For this review, take the finished solid that the model builds, in its own axes (mm). A direction names the side the tool comes from. Round coordinates to 2 decimals unless told otherwise and drop trailing zeros. Order: outer loops, then holes, each group sorted by start corner. A loop starts at its lowest first (then second) coordinate and runs counter-clockwise, first axis right, second up. Notation, with made-up numbers: (2, -15) -> (29, -15) arc R17 cw to (29, -5) -> close; hole circle Ø8 at (-40, 59). An arc over 180 degrees is marked (long way). Use a Markdown table: item, result. Add a question column.
1) Clearance check with flat-ended pins moving along their axes: P1, Ø7.5, axis at x = -22, y = -5, coming from the +Z side; P2, Ø3, axis at x = -6.5, y = -4.5, coming from the +Z side; P3, Ø1, axis at y = 10.5, z = -4, coming from the -X side; P4, Ø3, axis at y = -3, z = -4, coming from the -X side. State where each tip first meets the part, or that it passes through.
2) Consider section B-B (y = 21.5). State the section outline as (x, z) points, plus the area to 3 significant figures.
3) Wall thickness on line 1 along X through (y, z) = (11.5, -4.5); line 2 along Y through (x, z) = (8.3, 0); line 3 along Z through (x, y) = (-20, 21.5): over which ranges is each line inside the solid? List them lowest first. Write a range as [from, to].
4) Consider section A-A (y = 11). State the section outline as (x, z) points.
5) Draft analysis for pull direction Z (two halves, no side actions). For faces 5 (the face through (-7.5, 15, -4)), 6 (the face through (8.6, -18.8, -1.6)), 7 (the face through (-18, -1, 3.5)), state which applies: pulls with the +Z half, pulls with the -Z half, needs draft (parallel to the pull), parting line crosses it, or undercut.
6) Machinability: for faces 1 (the face through (1.4, 2.5, -4.5)), 2 (the face through (-16, 10, 4)), 3 (the face through (-26, 18, -3.5)), 4 (the face through (-18, -4, -3.5)), which of the approach directions +Z, -Z, +X, -X, +Y, -Y give a long, thin tool a straight path to every point of the face, cutting with its end or side? Answer none if there is none.
7) Consider section C-C (x = 3). State the section outline as (y, z) points, plus the area to 3 significant figures.
8) Consider section D-D (z = -6.25). State the section outline as (x, y) points, plus the area to 3 significant figures.
```python
from build123d import *

# Parameters (mm, degrees)
SKETCH2_R               = 10
BOSS_EXTRUDE1_DEPTH     = 30
CUT_EXTRUDE1_START      = -10
SKETCH3_R               = 10
SKETCH3_R_2             = 7.5
CUT_EXTRUDE1_DEPTH      = 10
CUT_EXTRUDE3_DEPTH      = 10
CUT_EXTRUDE3_DEPTH_BACK = 10
SKETCH5_R               = 2
FILLET2_R               = 10
BOSS_EXTRUDE2_START     = -67.5
SKETCH7_R               = 10
BOSS_EXTRUDE2_DEPTH     = 67.5
SKETCH8_R               = 50
SKETCH8_R_2             = 10
CUT_EXTRUDE6_DEPTH      = 107.770782567
SKETCH9_R               = 7.5
CUT_EXTRUDE7_DEPTH      = 10
CUT_EXTRUDE8_DEPTH      = 10
CUT_EXTRUDE8_DEPTH_BACK = 10
SKETCH10_R              = 2
CUT_EXTRUDE9_DEPTH      = 48
CUT_EXTRUDE9_DEPTH_BACK = 29
SKETCH12_W              = 23.028444079
SKETCH12_H              = 65
SKETCH13_W              = 45
SKETCH13_H              = 7
BOSS_EXTRUDE3_DEPTH     = 15
SKETCH14_W              = 7
SKETCH14_H              = 25.920736851
BOSS_EXTRUDE4_DEPTH     = 2
SKETCH15_W              = 17.5
SKETCH15_H              = 25.366229316
BOSS_EXTRUDE5_DEPTH     = 2
SKETCH15_W_2            = 16.786959534
BOSS_EXTRUDE5_2_DEPTH   = 2
BOSS_EXTRUDE6_START     = -44.28696
BOSS_EXTRUDE6_DEPTH     = 44.28696
SKETCH17_W              = 10
SKETCH17_H              = 2
SKETCH17_W_2            = 18.286959534
SKETCH17_W_3            = 19
CUT_EXTRUDE10_DEPTH     = 8
BOSS_EXTRUDE7_DEPTH     = 19.367497
CUT_EXTRUDE11_DEPTH     = 8
SKETCH22_W              = 1.1
SKETCH22_H              = 2
CUT_EXTRUDE12_DEPTH     = 32
SKETCH23_W              = 5.9
SKETCH23_H              = 12.960368426
CUT_EXTRUDE13_DEPTH     = 10


with BuildPart() as part:
    # Sketch1 → Revolve1 (revolve)
    with BuildSketch(Plane.XY):
        Polygon((50, 25), (0, 25), (0, 22.5), (45, 22.5), (45, -22.5), (0, -22.5), (0, -25), (50, -25), align=None)
    revolve(axis=Axis((0, -25, 0), (0, 1, 0)))

    # Sketch2 → Boss-Extrude1 (add)
    with BuildSketch(Plane(origin=(0, 25, 0), x_dir=(1, 0, 0), z_dir=(0, 1, 0))):
        with Locations(Location((0, 0, 0), (0, 0, 180))):
            Circle(SKETCH2_R)
    extrude(amount=BOSS_EXTRUDE1_DEPTH)

    # Sketch3 → Cut-Extrude1 (cut)
    with BuildSketch(Plane(origin=(0, 55, 0), x_dir=(1, 0, 0), z_dir=(0, 1, 0)).offset(CUT_EXTRUDE1_START)):
        with Locations(Location((0, 0, 0), (0, 0, 180))):
            Circle(SKETCH3_R)
        with Locations(Location((0, 0, 0), (0, 0, 180))):
            Circle(SKETCH3_R_2, mode=Mode.SUBTRACT)
    extrude(amount=CUT_EXTRUDE1_DEPTH, mode=Mode.SUBTRACT)

    # Sketch5 → Cut-Extrude3 (cut, two sides: drawn at the far end of the back side and taken through both)
    with BuildSketch(Plane(origin=(0, 0, 0), x_dir=(0, 0, -1), z_dir=(1, 0, 0)).offset(-CUT_EXTRUDE3_DEPTH_BACK)):
        with Locations(Location((0, 50, 0), (0, 0, 180))):
            Circle(SKETCH5_R)
    extrude(amount=CUT_EXTRUDE3_DEPTH + CUT_EXTRUDE3_DEPTH_BACK, mode=Mode.SUBTRACT)

    # Fillet2
    fillet2_edges = [part.edges().sort_by_distance(p)[0] for p in [
        (-50, 25, 0),
    ]]
    fillet(fillet2_edges, radius=FILLET2_R)

    # Sketch7 → Boss-Extrude2 (add)
    with BuildSketch(Plane(origin=(0, 45, 0), x_dir=(1, 0, 0), z_dir=(0, 1, 0)).offset(BOSS_EXTRUDE2_START)):
        with Locations(Location((0, 0, 0), (0, 0, 180))):
            Circle(SKETCH7_R)
    extrude(amount=BOSS_EXTRUDE2_DEPTH)

    # Sketch8 → Cut-Extrude6 (cut, through all)
    with BuildSketch(Plane(origin=(0, 55, 0), x_dir=(1, 0, 0), z_dir=(0, 1, 0))):
        Circle(SKETCH8_R)
        with Locations(Location((0, 0, 0), (0, 0, 180))):
            Circle(SKETCH8_R_2, mode=Mode.SUBTRACT)
    extrude(amount=-CUT_EXTRUDE6_DEPTH, mode=Mode.SUBTRACT)

    # Sketch9 → Cut-Extrude7 (cut)
    with BuildSketch(Plane.XZ.offset(25)):
        with Locations(Location((0, 0, 0), (0, 0, 180))):
            Circle(SKETCH9_R)
    extrude(amount=-CUT_EXTRUDE7_DEPTH, mode=Mode.SUBTRACT)

    # Sketch10 → Cut-Extrude8 (cut, two sides: drawn at the far end of the back side and taken through both)
    with BuildSketch(Plane(origin=(0, 0, 0), x_dir=(0, 0, -1), z_dir=(1, 0, 0)).offset(-CUT_EXTRUDE8_DEPTH_BACK)):
        with Locations(Location((0, -20, 0), (0, 0, 180))):
            Circle(SKETCH10_R)
    extrude(amount=CUT_EXTRUDE8_DEPTH + CUT_EXTRUDE8_DEPTH_BACK, mode=Mode.SUBTRACT)

    # Sketch12 → Cut-Extrude9 (cut, two sides: drawn at the far end of the back side and taken through both)
    with BuildSketch(Plane(origin=(0, 0, 0), x_dir=(0, 0, -1), z_dir=(1, 0, 0)).offset(-CUT_EXTRUDE9_DEPTH_BACK)):
        with Locations((0.475794299, 22.5)):
            Rectangle(SKETCH12_W, SKETCH12_H)
    extrude(amount=CUT_EXTRUDE9_DEPTH + CUT_EXTRUDE9_DEPTH_BACK, mode=Mode.SUBTRACT)

    # Sketch13 → Boss-Extrude3 (add)
    with BuildSketch(Plane(origin=(0, -10, 0), x_dir=(1, 0, 0), z_dir=(0, 1, 0))):
        with Locations((-12.5, 0)):
            Rectangle(SKETCH13_W, SKETCH13_H)
    extrude(amount=BOSS_EXTRUDE3_DEPTH)

    # Sketch14 → Boss-Extrude4 (add)
    with BuildSketch(Plane.XY.offset(3.5)):
        with Locations((-12.5, 17.264610389)):
            Rectangle(SKETCH14_W, SKETCH14_H)
    extrude(amount=BOSS_EXTRUDE4_DEPTH)



with BuildPart() as body_2:
    # Sketch15 → Boss-Extrude5 (new body)
    with BuildSketch(Plane(origin=(0, 0, -3.5), x_dir=(-1, 0, 0), z_dir=(0, 0, -1))):
        with Locations((-1.25, 17.683114658)):
            Rectangle(SKETCH15_W, SKETCH15_H)
    extrude(amount=BOSS_EXTRUDE5_DEPTH)


with BuildPart() as body_3:
    # Sketch15 → Boss-Extrude5 2 (new body)
    with BuildSketch(Plane(origin=(0, 0, -3.5), x_dir=(-1, 0, 0), z_dir=(0, 0, -1))):
        with Locations((25.893479767, 17.683114658)):
            Rectangle(SKETCH15_W_2, SKETCH15_H)
    extrude(amount=BOSS_EXTRUDE5_2_DEPTH)


with BuildPart() as part_1:
    add(part.part)

    add(body_2.part)  # Boss-Extrude6 merges body 2

    add(body_3.part)  # Boss-Extrude6 merges body 3
    # Sketch16 → Boss-Extrude6 (add)
    with BuildSketch(Plane.ZY.offset(34.286959534).offset(BOSS_EXTRUDE6_START)):
        Polygon((-5.5, 5), (-3.5, 0), (-3.5, 5), align=None)
        Polygon((3.5, 0), (5.5, 4.304241963), (3.5, 4.304241963), align=None)
    extrude(amount=BOSS_EXTRUDE6_DEPTH)

    # Sketch17 → Cut-Extrude10 (cut)
    with BuildSketch(Plane(origin=(0, 5, 0), x_dir=(1, 0, 0), z_dir=(0, 1, 0))):
        with Locations((-12.5, 4.5)):
            Rectangle(SKETCH17_W, SKETCH17_H)
        with Locations((-25.143479767, -4.5)):
            Rectangle(SKETCH17_W_2, SKETCH17_H)
        with Locations((0.5, -4.5)):
            Rectangle(SKETCH17_W_3, SKETCH17_H)
    extrude(amount=-CUT_EXTRUDE10_DEPTH, mode=Mode.SUBTRACT)

    # Sketch18 → Boss-Extrude7 (add)
    with BuildSketch(Plane(origin=(10, 0, 0), x_dir=(0, 0, -1), z_dir=(1, 0, 0))):
        Polygon((-10, -10), (-3.5, -10), (-3.5, -2.5), align=None)
        Polygon((10, -10), (3.5, -4.366666667), (3.5, -10), align=None)
    extrude(amount=-BOSS_EXTRUDE7_DEPTH)

    # Sketch19 → Cut-Extrude11 (cut)
    with BuildSketch(Plane.XZ.offset(10)):
        with BuildLine():
            ThreePointArc((0, 10), (7.071067812, 7.071067812), (10, 0))
            Line((10, 0), (10, 10))
            Line((10, 10), (0, 10))
        make_face()
        with BuildLine():
            Line((-13.702189606, 3.5), (-9.367496998, 3.5))
            ThreePointArc((-9.367496998, 3.5), (-5.700877125, 8.215838363), (0, 10))
            Line((0, 10), (10, 10))
            ThreePointArc((10, 10), (-3.740194109, 13.638583065), (-13.702189606, 3.5))
        make_face()
        with BuildLine():
            ThreePointArc((10, 0), (1.778346145, -9.840603893), (-9.367496998, -3.5))
            Line((-9.367496998, -3.5), (-13.702189606, -3.5))
            ThreePointArc((-13.702189606, -3.5), (6.999217954, -12.288651188), (10, 10))
            Line((10, 10), (10, 0))
        make_face()
    extrude(amount=-CUT_EXTRUDE11_DEPTH, mode=Mode.SUBTRACT)

    # Sketch22 → Cut-Extrude12 (cut)
    with BuildSketch(Plane(origin=(0, 30.224978814, 0), x_dir=(1, 0, 0), z_dir=(0, 1, 0))):
        with Locations((-9.55, -4.5)):
            Rectangle(SKETCH22_W, SKETCH22_H)
    extrude(amount=-CUT_EXTRUDE12_DEPTH, mode=Mode.SUBTRACT)

    # Sketch23 → Cut-Extrude13 (cut)
    with BuildSketch(Plane.XY.offset(5.5)):
        with Locations((-13.05, 23.744794601)):
            Rectangle(SKETCH23_W, SKETCH23_H)
    extrude(amount=-CUT_EXTRUDE13_DEPTH, mode=Mode.SUBTRACT)


solid = part_1.part
```
Results list:
| question | item | result |
|---|---|---|
| 1 | P1 | z = 3.5 |
| 1 | P2 | z = 6.53 |
| 1 | P3 | x = -34.29 |
| 1 | P4 | x = -35 |
| 2 | outline | (-34.29, -5.5) -> (-17.5, -5.5) -> (-17.5, -3.5) -> (-34.29, -3.5) -> close; (-7.5, -5.5) -> (10, -5.5) -> (10, -3.5) -> (-7.5, -3.5) -> close |
| 2 | area | 68.6 mm2 |
| 3 | line 1 | [-34.29, -17.5], [-7.5, 10] |
| 3 | line 2 | [-25, -22], [-18, 5] |
| 3 | line 3 | [-5.5, -3.5] |
| 4 | outline | (-34.29, -5.5) -> (-17.5, -5.5) -> (-17.5, -3.5) -> (-34.29, -3.5) -> close; (-16, 3.5) -> (-10.1, 3.5) -> (-10.1, 5.5) -> (-16, 5.5) -> close; (-7.5, -5.5) -> (10, -5.5) -> (10, -3.5) -> (-7.5, -3.5) -> close |
| 5 | face 5 | needs draft |
| 5 | face 6 | undercut |
| 5 | face 7 | pulls with the +Z half |
| 6 | face 1 | -Z, +X, -X |
| 6 | face 2 | +Z, -X, +Y, -Y |
| 6 | face 3 | +Z, +X, -X, +Y |
| 6 | face 4 | -Z |
| 7 | outline | (-25, -9.54) -> (-9.6, -9.54) -> (-4.37, -3.5) -> (0, -3.5) -> (5, -5.5) -> (30.37, -5.5) -> (30.37, -3.5) -> (5, -3.5) -> (5, 3.5) -> (-2.5, 3.5) -> (-9.47, 9.54) -> (-25, 9.54) -> (-25, 6.87) -> (-15, 6.87) -> (-15, -6.87) -> (-25, -6.87) -> close |
| 7 | area | 352 mm2 |
| 8 | outline | (-7.81, -25) -> (-4.15, -25) -> (-4.15, -15) -> (4.15, -15) -> (4.15, -25) -> (7.81, -25) -> (7.81, -6.75) -> (-7.81, -6.75) -> close |
| 8 | area | 202 mm2 |
